from build123d import *

# Parameters (mm, degrees)
BOSS_EXTRUDE1_DEPTH = 40
BOSS_EXTRUDE2_START = 40
BOSS_EXTRUDE2_DEPTH = 4
SKETCH3_R           = 1.7
BOSS_EXTRUDE3_DEPTH = 4
CUT_EXTRUDE1_DEPTH  = 4
SKETCH5_W           = 4
SKETCH5_H           = 44
CUT_EXTRUDE2_DEPTH  = 30
SKETCH6_R           = 2
CUT_EXTRUDE3_DEPTH  = 93.173748974
FILLET1_R           = 5


with BuildPart() as part:
    # Sketch1 → Boss-Extrude1 (new body)
    with BuildSketch(Plane(origin=(0, 0, 0), x_dir=(1, 0, 0), z_dir=(0, 1, 0))):
        with BuildLine():
            Line((-35, 28), (35, 28))
            ThreePointArc((35, 28), (63, 0), (35, -28))
            Line((35, -28), (-35, -28))
            ThreePointArc((-35, -28), (-63, 0), (-35, 28))
        make_face()
        with BuildLine():
            Line((-35, 25), (35, 25))
            ThreePointArc((35, 25), (60, 0), (35, -25))
            Line((35, -25), (-35, -25))
            ThreePointArc((-35, -25), (-60, 0), (-35, 25))
        make_face(mode=Mode.SUBTRACT)
    extrude(amount=BOSS_EXTRUDE1_DEPTH)

    # Sketch1<2> → Boss-Extrude2 (add)
    with BuildSketch(Plane(origin=(0, 0, 0), x_dir=(1, 0, 0), z_dir=(0, 1, 0)).offset(BOSS_EXTRUDE2_START)):
        with BuildLine():
            Line((-35, 28), (35, 28))
            ThreePointArc((35, 28), (63, 0), (35, -28))
            Line((35, -28), (-35, -28))
            ThreePointArc((-35, -28), (-63, 0), (-35, 28))
        make_face()
    extrude(amount=BOSS_EXTRUDE2_DEPTH)

    # Sketch3 → Boss-Extrude3 (add)
    with BuildSketch(Plane.XZ):
        with BuildLine():
            Line((-62.549954628, 5), (-71, 5))
            ThreePointArc((-71, 5), (-76, 0), (-71, -5))
            Line((-71, -5), (-62.549954628, -5))
            ThreePointArc((-62.549954628, -5), (-63, 0), (-62.549954628, 5))
        make_face()
        with Locations(Location((-71, 0, 0), (0, 0, 270))):
            Circle(SKETCH3_R, mode=Mode.SUBTRACT)
    boss_extrude3 = extrude(amount=-BOSS_EXTRUDE3_DEPTH)

    # Mirror1: Boss-Extrude3 across plane
    add(boss_extrude3.mirror(Plane(origin=(0, 0, 0), x_dir=(0, 0, 1), z_dir=(1, 0, 0))))

    # Sketch4 → Cut-Extrude1 (cut)
    with BuildSketch(Plane(origin=(0, 0, 25), x_dir=(-1, 0, 0), z_dir=(0, 0, -1))):
        with BuildLine():
            Line((6, 10), (6, 0))
            Line((6, 0), (-6, 0))
            Line((-6, 0), (-6, 10))
            ThreePointArc((-6, 10), (0, 16), (6, 10))
        make_face()
    extrude(amount=-CUT_EXTRUDE1_DEPTH, mode=Mode.SUBTRACT)

    # Sketch5 → Cut-Extrude2 (cut)
    with BuildSketch(Plane.XY.offset(28)):
        with Locations((0, 22)):
            Rectangle(SKETCH5_W, SKETCH5_H)
    extrude(amount=-CUT_EXTRUDE2_DEPTH, mode=Mode.SUBTRACT)

    # Sketch6 → Cut-Extrude3 (cut, through all)
    with BuildSketch(Plane(origin=(0, 44, 0), x_dir=(1, 0, 0), z_dir=(0, 1, 0))):
        with Locations((0, 2)):
            Circle(SKETCH6_R)
    extrude(amount=-CUT_EXTRUDE3_DEPTH, mode=Mode.SUBTRACT)

    # Fillet1
    fillet1_edges = [part.edges().sort_by_distance(p)[0] for p in [
        (18.5, 44, 28),
        (-63, 44, 0),
        (0, 44, -28),
        (63, 44, 0),
    ]]
    fillet(fillet1_edges, radius=FILLET1_R)


solid = part.part
Can you work these out from the model? Positions are in its coordinate system, mm. A direction names the side the tool comes from. Give positions to 0.01 mm unless a question says otherwise; leave off trailing zeros. Write each loop counter-clockwise with the first axis right and the second up, starting at its lowest first coordinate (ties: lowest second). Pieces come first, ordered by that corner, then holes. Notation, with made-up numbers: M 36.5,-16 L 40.5,-16 A25 cw 40.5,-3 Z; hole C 38.5,-17.5 d3. An arc over 180 degrees is marked long. Answer in a Markdown table with one row per item. Add a question column.
Item 1: Imagine slicing it at A-A, the plane z = 0. Write out the boundary of the cut face in (x, y), plus the area to 3 significant figures.
Item 2: Please list where these lines run through material, in increasing order: L1, parallel to X at y = 1.4, z = 0; L2, parallel to Z at x = 71, y = 3; L3, parallel to Z at x = 35, y = 35.5.
Item 3: On a 3-axis mill with a long thin cutter (end or side, diameter ignored), from which of +Z, -Z, +X, -X, +Y, -Y can I reach the whole of each face in a straight line? I mean faces 1 (the flat face through (-6, 5, 26)), 2 (the flat face through (0, 20, -25)), 3 (the flat face through (2, 40.3, 17.5)), 4 (the flat face through (-67, 2, 5)). Say none if no direction works.
Item 4: Imagine slicing it at C-C, the plane y = 8. Write out the boundary of the cut face in (x, z).
Item 5: Imagine slicing it at B-B, the plane y = 20.5. Write out the boundary of the cut face in (x, z), plus the area to 3 significant figures.
Item 6: We'd pull the mould along Z, two halves only. Please class faces 5 (the cylindrical face through (76, 2, 0)), 6 (the flat face through (19, 20, 25)), 7 (the flat face through (67, 2, 5)): released by +Z, released by -Z, zero draft, split by the parting line, or undercut.
Item 7: For pin 1 Ø22.5 at (y, z) = (30, 7) entering from +X; pin 2 Ø25 at (x, z) = (-8.5, -10) entering from -Y; pin 3 Ø5 at (x, z) = (68.5, 1.5) entering from +Y, each with a flat end and sliding along its axis, tell me the tip position at first contact or that it passes through.
Evaluation:
| question | item | result |
|---|---|---|
| 1 | outline | M -76,0 L -72.7,0 L -72.7,4 L -76,4 Z; M -69.3,0 L -60,0 L -60,40 L -2,40 L -2,44 L -58,44 A5 ccw -63,39 L -63,4 L -69.3,4 Z; M 2,40 L 60,40 L 60,0 L 69.3,0 L 69.3,4 L 63,4 L 63,39 A5 ccw 58,44 L 2,44 Z; M 72.7,0 L 76,0 L 76,4 L 72.7,4 Z |
| 1 | area | 794 mm² |
| 2 | L1 | x = -76 to -72.7, -69.3 to -60, 60 to 69.3, 72.7 to 76 |
| 2 | L2 | z = -5 to -1.7, 1.7 to 5 |
| 2 | L3 | z = -28 to -25, 25 to 28 |
| 3 | face 1 | +Z, -Y |
| 3 | face 2 | -Y |
| 3 | face 3 | +Z, +Y, -Y |
| 3 | face 4 | +Z, -X, +Y, -Y |
| 4 | outline | M -35,-28 L 35,-28 A28 ccw 35,28 L 6,28 L 6,25 L 35,25 A25 cw 35,-25 L -35,-25 A25 cw -35,25 L -6,25 L -6,28 L -35,28 A28 ccw Z |
| 5 | outline | M -35,-28 L 35,-28 A28 ccw 35,28 L 2,28 L 2,25 L 35,25 A25 cw 35,-25 L -35,-25 A25 cw -35,25 L -2,25 L -2,28 L -35,28 A28 ccw Z |
| 5 | area | 908 mm² |
| 6 | face 5 | split by the parting line |
| 6 | face 6 | undercut |
| 6 | face 7 | released by +Z |
| 7 | pin 1 | stops at x = 63 |
| 7 | pin 2 | stops at y = 40 |
| 7 | pin 3 | stops at y = 4 |
